The listing builds one solid part. Answer for the finished solid, in the listing's coordinates (mm). Face numbers are marked on the shaded views. A direction names the side the tool comes from. Round coordinates to 2 decimals unless told otherwise and drop trailing zeros. Order: outer loops, then holes, each group sorted by start corner. A loop starts at its lowest first (then second) coordinate and runs counter-clockwise, first axis right, second up. Notation, with made-up numbers: M 11,-11 L 27,-11 A12 cw 27,-7 Z; hole C 10.25,52.5 d11. An arc over 180 degrees is marked long. Write item = value, one per line. Start each with the question number.
(1) Straight lines are drawn through the part: probe 1 along Y at (x, z) = (0, 0.3); probe 2 along Y at (x, z) = (-1, 4.5); probe 3 along X at (y, z) = (2, 5.5). For each, find the intervals that lie inside material, in ascending order. Write a range as from..to.
(2) A cutting plane is placed at D-D, the plane z = 1. Determine the outline of the cut face in (x, y).
(3) A cutting plane is placed at B-B, the plane z = 11.5. Determine the outline of the cut face in (x, y), and give its area (3 significant figures).
(4) Which of the six approach directions +Z, -Z, +X, -X, +Y, -Y give full straight-line access (tool end or side, diameter ignored) to the marked faces 4, 5 and 6?
(5) A cutting plane is placed at A-A, the plane y = 0. Determine the outline of the cut face in (x, z) (3 decimals), and give its area (3 significant figures).
(6) Each of these flat-tipped pins is pushed along its axis until it touches: pin 1 (1.5 mm diameter, centred on x = 4.5, z = 9.5, fed in from -Y); pin 2 (1.5 mm diameter, centred on x = -4.5, y = -4.5, fed in from -Z) (3 decimals); pin 3 (2.5 mm diameter, centred on x = 2, y = 1, fed in from +Z). Where does it stop, or does it pass through?
(7) A cutting plane is placed at C-C, the plane y = -4.5. Determine the outline of the cut face in (x, z) (3 decimals), and give its area (3 significant figures).
(8) For a pull along Y with two mould halves and no side action, classify the marked faces 1, 2 and 3 as released by +Y, released by -Y, zero draft, split by the parting line, or undercut.
from build123d import *

# Parameters (mm, degrees)
BOSS_EXTRUDE1_DEPTH         = 11.811
SKETCH5_R                   = 5.461
BOSS_EXTRUDE3_DEPTH         = 3.5306
F_3_8_24_TAPPED_HOLE2_D     = 8.4328
F_3_8_24_TAPPED_HOLE2_DEPTH = 12.065
F_3_8_24_TAPPED_HOLE2_TIP   = 2.533468714
SKETCH9_R                   = 3.07975
CUT_EXTRUDE1_DEPTH          = 16.3416
SKETCH10_R                  = 4.1529
CUT_EXTRUDE2_DEPTH          = 4.445
SKETCH11_OUTSIDE_W          = 17.688
SKETCH11_OUTSIDE_H          = 19.408
SKETCH11_OUTSIDE_R          = 5.461
CUT_EXTRUDE3_DEPTH          = 1.905


with BuildPart() as part:
    # Sketch1 → Boss-Extrude1 (new body)
    with BuildSketch(Plane.XY):
        Polygon((5.55625, -3.207902433), (5.55625, 3.207902433), (0, 6.415804866), (-5.55625, 3.207902433), (-5.55625, -3.207902433), (0, -6.415804866), align=None)
    extrude(amount=BOSS_EXTRUDE1_DEPTH)

    # Sketch5 → Boss-Extrude3 (add)
    with BuildSketch(Plane.XY.offset(11.811)):
        Circle(SKETCH5_R)
    extrude(amount=BOSS_EXTRUDE3_DEPTH)

    # 3/8-24 Tapped Hole2
    with Locations(Plane.XY.offset(15.3416)):
        with Locations((0, 0)):
            Hole(F_3_8_24_TAPPED_HOLE2_D / 2, depth=F_3_8_24_TAPPED_HOLE2_DEPTH)
            with Locations((0, 0, -(F_3_8_24_TAPPED_HOLE2_DEPTH + F_3_8_24_TAPPED_HOLE2_TIP / 2))):  # 118° drill point
                Cone(0, F_3_8_24_TAPPED_HOLE2_D / 2, F_3_8_24_TAPPED_HOLE2_TIP, mode=Mode.SUBTRACT)

    # Sketch9 → Cut-Extrude1 (cut, through all)
    with BuildSketch(Plane(origin=(0, 0, 0), x_dir=(-1, 0, 0), z_dir=(0, 0, -1))):
        Circle(SKETCH9_R)
    extrude(amount=-CUT_EXTRUDE1_DEPTH, mode=Mode.SUBTRACT)

    # Sketch10 → Cut-Extrude2 (cut)
    with BuildSketch(Plane.XY.offset(5.8166)):
        Circle(SKETCH10_R)
    extrude(amount=-CUT_EXTRUDE2_DEPTH, mode=Mode.SUBTRACT)

    # Sketch11 outside → Cut-Extrude3 (cut)
    with BuildSketch(Plane(origin=(0, 0, 0), x_dir=(-1, 0, 0), z_dir=(0, 0, -1))):
        Rectangle(SKETCH11_OUTSIDE_W, SKETCH11_OUTSIDE_H)
        with Locations(Location((0, 0, 0), (0, 0, 180))):  # turned: the seam where the file's is
            Circle(SKETCH11_OUTSIDE_R, mode=Mode.SUBTRACT)
    extrude(amount=-CUT_EXTRUDE3_DEPTH, mode=Mode.SUBTRACT)


solid = part.part
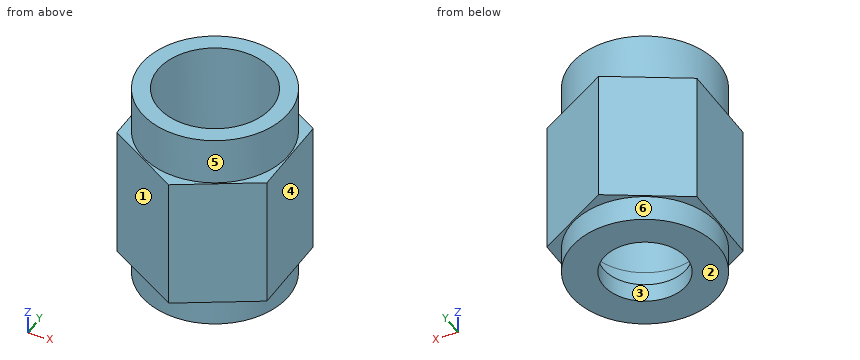
Reported:
q1.probe_1 = -5.46..-3.08, 3.08..5.46
q1.probe_2 = -5.84..-4.1, 4.1..5.84
q1.probe_3 = -5.56..-3.71, 3.71..5.56
q2.outline = C 0,0 d10.92; hole C 0,0 d6.16
q3.outline = M -5.56,-3.21 L 0,-6.42 L 5.56,-3.21 L 5.56,3.21 L 0,6.42 L -5.56,3.21 Z; hole C 0,0 d8.43
q3.area = 51.1 mm²
q4.face_4 = +Z, -Z, +X, +Y, -Y
q4.face_5 = +Z
q4.face_6 = -Z
q5.outline = M -5.556,1.905 L -5.461,1.905 L -5.461,0 L -3.08,0 L -3.08,1.372 L -4.153,1.372 L -4.153,3.238 L -4.216,3.277 L -4.216,15.342 L -5.461,15.342 L -5.461,11.811 L -5.556,11.811 Z; M 3.08,0 L 5.461,0 L 5.461,1.905 L 5.556,1.905 L 5.556,11.811 L 5.461,11.811 L 5.461,15.342 L 4.216,15.342 L 4.216,3.277 L 4.153,3.238 L 4.153,1.372 L 3.08,1.372 Z
q5.area = 43.4 mm²
q6.pin_1 = -4.25
q6.pin_2 = 1.905
q6.pin_3 = 1.37
q7.outline = M -3.318,1.905 L -3.094,1.905 L -3.094,0 L 3.094,0 L 3.094,1.905 L 3.318,1.905 L 3.318,11.811 L 3.094,11.811 L 3.094,15.342 L -3.094,15.342 L -3.094,11.811 L -3.318,11.811 Z
q7.area = 99.4 mm²
q8.face_1 = released by -Y
q8.face_2 = zero draft
q8.face_3 = undercut
